from build123d import *

# Parameters (mm, degrees)
SKETCH1_W                  = 355.6
SKETCH1_H                  = 770.128
BOSS_EXTRUDE1_DEPTH        = 3.175
F_1_1_DIAMETER_HOLE1_D     = 25.4
F_1_1_DIAMETER_HOLE1_DEPTH = 20.574
F_1_1_DIAMETER_HOLE1_TIP   = 7.630929862
SKETCH4_R                  = 11.1125
CUT_EXTRUDE1_DEPTH         = 4.175


with BuildPart() as part:
    # Sketch1 → Boss-Extrude1 (new body)
    with BuildSketch(Plane(origin=(0, 0, 0), x_dir=(1, 0, 0), z_dir=(0, 1, 0))):
        with Locations((177.8, 385.064)):
            Rectangle(SKETCH1_W, SKETCH1_H)
    extrude(amount=BOSS_EXTRUDE1_DEPTH)

    # 1 (1) Diameter Hole1
    with Locations(Plane(origin=(0, 3.175, 0), x_dir=(-1, 0, 0), z_dir=(0, 1, 0))):
        with Locations((-50.8, -38.1), (-50.8, -732.028), (-304.8, -732.028), (-304.8, -38.1)):
            Hole(F_1_1_DIAMETER_HOLE1_D / 2, depth=F_1_1_DIAMETER_HOLE1_DEPTH)
            with Locations((0, 0, -(F_1_1_DIAMETER_HOLE1_DEPTH + F_1_1_DIAMETER_HOLE1_TIP / 2))):  # 118° drill point
                Cone(0, F_1_1_DIAMETER_HOLE1_D / 2, F_1_1_DIAMETER_HOLE1_TIP, mode=Mode.SUBTRACT)

    # Sketch4 → Cut-Extrude1 (cut, through all)
    with BuildSketch(Plane(origin=(0, 3.175, 0), x_dir=(1, 0, 0), z_dir=(0, 1, 0))):
        with Locations((127, 38.1)):
            Circle(SKETCH4_R)
    extrude(amount=-CUT_EXTRUDE1_DEPTH, mode=Mode.SUBTRACT)


solid = part.part
Geometry check sheet. Reference: the model listing, model coordinates, mm. Coordinates: 2 decimals unless noted, no trailing zeros. Order: outer loops, then holes, each group sorted by start corner. A loop starts at its lowest first (then second) coordinate and runs counter-clockwise, first axis right, second up. Notation, with made-up numbers: M 76,-13 L 98,-13 A34 ccw 98,17 Z; hole C 19.25,-37.75 d2. An arc over 180 degrees is marked long. Use CSV: the item, a comma, the result in double quotes.
Item 1: Cross-section at B-B on x = 304.8. Record the cut outline in (y, z) (3 decimals), then the cut area to 3 significant figures.
Returned:
outline,"M 0,-770.128 L 3.175,-770.128 L 3.175,-744.728 L 0,-744.728 Z; M 0,-719.328 L 3.175,-719.328 L 3.175,-50.8 L 0,-50.8 Z; M 0,-25.4 L 3.175,-25.4 L 3.175,0 L 0,0 Z"
area,"2,280 mm2"
Item 2: Gauge pin test, flat ends, axial feed: pin 1 Ø20.5 at (x, z) = (50.8, -38.1) entering from +Y; pin 2 Ø1.5 at (x, z) = (305.5, -684) entering from -Y. Record the tip position at first contact, or that the pin passes through.
Returned:
pin 1,"passes through"
pin 2,"stops at y = 0"
Item 3: Mould release check, pull along X, two halves, no side actions. Record for faces 1 (the cylindrical face through (115.9, 1.6, -38.6)), 2 (the flat face through (175, 0, -390)), 3 (the cylindrical face through (302.047, 1.565, -744.426)): pulls with the +X half, pulls with the -X half, needs draft (parallel to the pull), parting line crosses it, or undercut.
Returned:
face 1,"undercut"
face 2,"needs draft"
face 3,"undercut"
Item 4: Cross-section at C-C on z = -38.1. Record the cut outline in (x, y) (1 decimal).
Returned:
outline,"M 0,0 L 38.1,0 L 38.1,3.2 L 0,3.2 Z; M 63.5,0 L 115.9,0 L 115.9,3.2 L 63.5,3.2 Z; M 138.1,0 L 292.1,0 L 292.1,3.2 L 138.1,3.2 Z; M 317.5,0 L 355.6,0 L 355.6,3.2 L 317.5,3.2 Z"
Item 5: Thickness scan on line 1 along Z through (x, y) = (50.8, 1.3); line 2 along X through (y, z) = (0.45, -732); line 3 along Z through (x, y) = (127, 1.55). Record the ranges inside material, lowest first.
Returned:
line 1,"z = -770.13 to -744.73, -719.33 to -50.8, -25.4 to 0"
line 2,"x = 0 to 38.1, 63.5 to 292.1, 317.5 to 355.6"
line 3,"z = -770.13 to -49.21, -26.99 to 0"
Item 6: Cross-section at A-A on x = 127. Record the cut outline in (y, z) (1 decimal), then the cut area to 3 significant figures.
Returned:
outline,"M 0,-770.1 L 3.2,-770.1 L 3.2,-49.2 L 0,-49.2 Z; M 0,-27 L 3.2,-27 L 3.2,0 L 0,0 Z"
area,"2,370 mm2"
